Work out the finished part from the listing and answer in its coordinate system (mm). Round coordinates to 2 decimals unless told otherwise and drop trailing zeros. Write each loop counter-clockwise with the first axis right and the second up, starting at its lowest first coordinate (ties: lowest second). Pieces come first, ordered by that corner, then holes. Notation, with made-up numbers: (-26, 73) - (-18, 73) arc R27 cw to (-18, 97) - close; hole circle Ø9 at (-4, 4). An arc over 180 degrees is marked (long way). Answer as a JSON object with one key per item and string values.
```python
from build123d import *

# Parameters (mm, degrees)
SKETCH1_W           = 210
SKETCH1_H           = 50
SKETCH1_R           = 1.211665018
SKETCH1_R_2         = 1.165617118
SKETCH1_R_3         = 1.5
SKETCH1_R_4         = 1.25
SKETCH1_R_5         = 1.517273905
SKETCH1_R_6         = 3.4
BOSS_EXTRUDE1_DEPTH = 3.175
SKETCH2_R           = 2
CUT_EXTRUDE1_DEPTH  = 10
SKETCH3_R           = 6
SKETCH3_R_2         = 0.586995366
CUT_EXTRUDE2_DEPTH  = 57.15
CUT_EXTRUDE7_DEPTH  = 10
FILLET3_R           = 5
SKETCH11_R          = 18.5
SKETCH11_R_2        = 2
BOSS_EXTRUDE4_DEPTH = 3.175
SKETCH16_W          = 18.257640281
SKETCH16_H          = 3.175
BOSS_EXTRUDE7_DEPTH = 8.128
SKETCH17_W          = 33.3
SKETCH17_H          = 3.175
BOSS_EXTRUDE8_DEPTH = 35.56
SKETCH18_R          = 2
CUT_EXTRUDE8_DEPTH  = 9
SKETCH19_R          = 4
CUT_EXTRUDE9_DEPTH  = 40
FILLET4_R           = 5
SKETCH20_R          = 3.5
CUT_EXTRUDE10_DEPTH = 10
SKETCH21_R          = 1.5
CUT_EXTRUDE11_DEPTH = 10
SKETCH22_R          = 1.5
CUT_EXTRUDE12_DEPTH = 10
SKETCH24_R          = 1.5
CUT_EXTRUDE13_DEPTH = 10
SKETCH25_W          = 49.782255358
SKETCH25_H          = 46.410966041
CUT_EXTRUDE14_DEPTH = 10


with BuildPart() as part:
    # Sketch1 → Boss-Extrude1 (new body)
    with BuildSketch(Plane(origin=(0, 0, 0), x_dir=(1, 0, 0), z_dir=(0, 1, 0))):
        with Locations((105, -25)):
            Rectangle(SKETCH1_W, SKETCH1_H)
        with Locations(Location((3.489526233, -16.787661112, 0), (0, 0, 270))):
            Circle(SKETCH1_R, mode=Mode.SUBTRACT)
        with Locations(Location((34.37258772, -17.194005245, 0), (0, 0, 270))):
            Circle(SKETCH1_R_2, mode=Mode.SUBTRACT)
        with Locations(Location((37.520749958, -44.921198121, 0), (0, 0, 270))):
            Circle(SKETCH1_R_3, mode=Mode.SUBTRACT)
        with Locations(Location((122, -42.058139805, 0), (0, 0, 270))):
            Circle(SKETCH1_R_4, mode=Mode.SUBTRACT)
        with Locations(Location((168.975233936, -37.403209633, 0), (0, 0, 270))):
            Circle(SKETCH1_R_5, mode=Mode.SUBTRACT)
        with Locations(Location((18, -34, 0), (0, 0, 270))):
            Circle(SKETCH1_R_6, mode=Mode.SUBTRACT)
    extrude(amount=BOSS_EXTRUDE1_DEPTH)

    # Sketch2 → Cut-Extrude1 (cut)
    with BuildSketch(Plane(origin=(0, 3.175, 0), x_dir=(1, 0, 0), z_dir=(0, 1, 0))):
        with Locations(Location((10, -26, 0), (0, 0, 270))):
            Circle(SKETCH2_R)
        with Locations(Location((10, -42, 0), (0, 0, 270))):
            Circle(SKETCH2_R)
        with Locations(Location((26, -26, 0), (0, 0, 270))):
            Circle(SKETCH2_R)
        with Locations(Location((26, -42, 0), (0, 0, 270))):
            Circle(SKETCH2_R)
    extrude(amount=-CUT_EXTRUDE1_DEPTH, mode=Mode.SUBTRACT)

    # Sketch3 → Cut-Extrude2 (cut)
    with BuildSketch(Plane(origin=(0, 3.175, 0), x_dir=(1, 0, 0), z_dir=(0, 1, 0))):
        with Locations(Location((78.01026379, -28.1, 0), (0, 0, 270))):
            Circle(SKETCH3_R)
        with Locations(Location((145.531297368, -14, 0), (0, 0, 270))):
            Circle(SKETCH3_R)
        with Locations((18, -34)):
            Circle(SKETCH3_R_2)
        with Locations(Location((202.646291021, -16, 0), (0, 0, 270))):
            Circle(SKETCH3_R)
    extrude(amount=-CUT_EXTRUDE2_DEPTH, mode=Mode.SUBTRACT)

    # Sketch10 → Cut-Extrude7 (cut)
    with BuildSketch(Plane(origin=(0, 3.175, 0), x_dir=(1, 0, 0), z_dir=(0, 1, 0))):
        Polygon((210, -27.859435908), (165.502877994, -50), (210, -50), align=None)
        Polygon((92.532613397, 0), (77.65477062, -7.402812063), (0, -7.402812063), (0, 0), align=None)
    extrude(amount=-CUT_EXTRUDE7_DEPTH, mode=Mode.SUBTRACT)

    # Fillet3
    fillet3_edges = [part.edges().sort_by_distance(p)[0] for p in [
        (210, 1.5875, 0),
        (92.532613397, 1.5875, 0),
        (210, 1.5875, 27.859435908),
        (165.502877994, 1.5875, 50),
        (77.65477062, 1.5875, 7.402812063),
    ]]
    fillet(fillet3_edges, radius=FILLET3_R)

    # Sketch11 → Boss-Extrude4 (add)
    with BuildSketch(Plane(origin=(0, 3.175, 0), x_dir=(1, 0, 0), z_dir=(0, 1, 0))):
        with Locations((18, -34)):
            Circle(SKETCH11_R)
        with Locations(Location((10, -26, 0), (0, 0, 270))):
            Circle(SKETCH11_R_2, mode=Mode.SUBTRACT)
        with Locations(Location((10, -42, 0), (0, 0, 270))):
            Circle(SKETCH11_R_2, mode=Mode.SUBTRACT)
        with Locations(Location((26, -26, 0), (0, 0, 270))):
            Circle(SKETCH11_R_2, mode=Mode.SUBTRACT)
        with Locations(Location((26, -42, 0), (0, 0, 270))):
            Circle(SKETCH11_R_2, mode=Mode.SUBTRACT)
    extrude(amount=-BOSS_EXTRUDE4_DEPTH)

    # Sketch16 → Boss-Extrude7 (add)
    with BuildSketch(Plane(origin=(0, 0, 7.402812063), x_dir=(-1, 0, 0), z_dir=(0, 0, -1))):
        with Locations((-9.128820141, 1.5875)):
            Rectangle(SKETCH16_W, SKETCH16_H)
    extrude(amount=BOSS_EXTRUDE7_DEPTH)

    # Sketch17 → Boss-Extrude8 (add)
    with BuildSketch(Plane.ZY):
        with Locations((15.924812063, 1.5875)):
            Rectangle(SKETCH17_W, SKETCH17_H)
    extrude(amount=BOSS_EXTRUDE8_DEPTH)

    # Sketch18 → Cut-Extrude8 (cut)
    with BuildSketch(Plane(origin=(0, 3.175, 0), x_dir=(1, 0, 0), z_dir=(0, 1, 0))):
        with Locations(Location((-29.612034681, -23.798543698, 0), (0, 0, 270))):
            Circle(SKETCH18_R)
        with Locations(Location((-29.359661767, -7.798707515, 0), (0, 0, 270))):
            Circle(SKETCH18_R)
        with Locations(Location((-13.359825583, -8.051080428, 0), (0, 0, 270))):
            Circle(SKETCH18_R)
        with Locations(Location((-13.612198497, -24.050916612, 0), (0, 0, 270))):
            Circle(SKETCH18_R)
    extrude(amount=-CUT_EXTRUDE8_DEPTH, mode=Mode.SUBTRACT)

    # Sketch19 → Cut-Extrude9 (cut)
    with BuildSketch(Plane(origin=(0, 3.175, 0), x_dir=(1, 0, 0), z_dir=(0, 1, 0))):
        with Locations(Location((-21.359661767, -15.798707515, 0), (0, 0, 270))):
            Circle(SKETCH19_R)
    extrude(amount=-CUT_EXTRUDE9_DEPTH, mode=Mode.SUBTRACT)

    # Fillet4
    fillet4_edges = [part.edges().sort_by_distance(p)[0] for p in [
        (18.257640281, 1.5875, -0.725187937),
        (-35.56, 1.5875, -0.725187937),
        (-35.56, 1.5875, 32.574812063),
        (0, 1.5875, 50),
    ]]
    fillet(fillet4_edges, radius=FILLET4_R)

    # Sketch20 → Cut-Extrude10 (cut)
    with BuildSketch(Plane(origin=(0, 3.175, 0), x_dir=(1, 0, 0), z_dir=(0, 1, 0))):
        with Locations(Location((18, -34, 0), (0, 0, 270))):
            Circle(SKETCH20_R)
    extrude(amount=-CUT_EXTRUDE10_DEPTH, mode=Mode.SUBTRACT)

    # Sketch21 → Cut-Extrude11 (cut)
    with BuildSketch(Plane(origin=(0, 3.175, 0), x_dir=(1, 0, 0), z_dir=(0, 1, 0))):
        with Locations(Location((116, -4.237214774, 0), (0, 0, 270))):
            Circle(SKETCH21_R)
    extrude(amount=-CUT_EXTRUDE11_DEPTH, mode=Mode.SUBTRACT)

    # Sketch22 → Cut-Extrude12 (cut)
    with BuildSketch(Plane(origin=(0, 3.175, 0), x_dir=(1, 0, 0), z_dir=(0, 1, 0))):
        with Locations(Location((12.257640281, -3.274812063, 0), (0, 0, 270))):
            Circle(SKETCH22_R)
    extrude(amount=-CUT_EXTRUDE12_DEPTH, mode=Mode.SUBTRACT)

    # Sketch24 → Cut-Extrude13 (cut)
    with BuildSketch(Plane(origin=(0, 3.175, 0), x_dir=(1, 0, 0), z_dir=(0, 1, 0))):
        with Locations(Location((-30.56, -15.774812063, 0), (0, 0, 270))):
            Circle(SKETCH24_R)
    extrude(amount=-CUT_EXTRUDE13_DEPTH, mode=Mode.SUBTRACT)

    # Sketch25 → Cut-Extrude14 (cut)
    with BuildSketch(Plane(origin=(0, 3.175, 0), x_dir=(1, 0, 0), z_dir=(0, 1, 0))):
        with Locations((-25.336149754, -9.369329043)):
            Rectangle(SKETCH25_W, SKETCH25_H)
    extrude(amount=-CUT_EXTRUDE14_DEPTH, mode=Mode.SUBTRACT)


solid = part.part
```
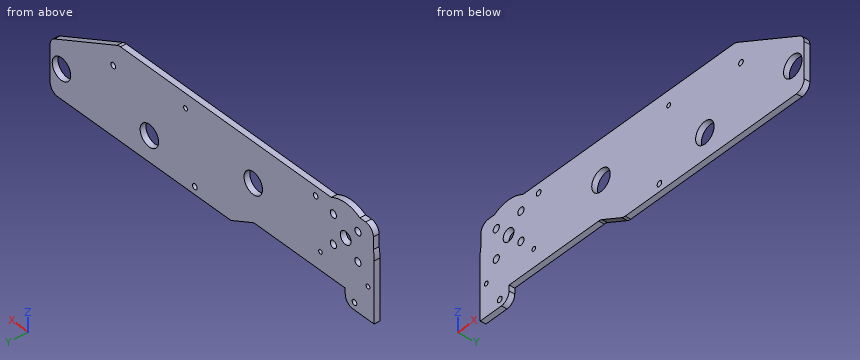
Item 1: A cutting plane is placed at B-B (y = 1.95). Give the number of separate pieces and of enclosed holes in the cut face, and give its area (3 significant figures).
Results found:
{"separate pieces": "1", "enclosed holes": "15", "area": "9,090 mm²"}
Item 2: A cutting plane is placed at A-A (x = 130.5). Write down the section's boundary in (y, z) (3 decimals), and give its area (3 significant figures).
Results found:
{"outline": "(0, 0) - (3.175, 0) - (3.175, 50) - (0, 50) - close", "area": "159 mm²"}
Item 3: Consider line 1 along X through (y, z) = (0.65, 41); line 2 along X through (y, z) = (0.95, 37); line 3 along Z through (x, y) = (103, 0.7). Determine where each line is inside the solid, lowest interval first.
Results found:
{"line 1": "0 to 8.27, 11.73 to 24.27, 27.73 to 121.33, 122.67 to 183.59", "line 2": "-0.26 to 16.2, 19.8 to 167.51, 170.44 to 191.63", "line 3": "0 to 50"}
Item 4: A cutting plane is placed at C-C (x = 50.5). Write down the section's boundary in (y, z) (3 decimals).
Results found:
{"outline": "(0, 7.403) - (3.175, 7.403) - (3.175, 50) - (0, 50) - close"}
Item 5: Each of these flat-tipped pins is pushed along its axis until it touches: P1, Ø1.8, axis at x = 12.26, z = 3.27, coming from the +Y side (3 decimals); P2, Ø1, axis at x = 6.5, y = 1.5, coming from the +Z side; P3, Ø1, axis at x = 163, y = 1.5, coming from the -Z side. Where does it stop, or does it pass through?
Results found:
{"P1": "through", "P2": "z = 50", "P3": "z = 0"}
